CAD build for the part. Positions are in the model's coordinates, mm. Face numbers are marked on the shaded views. Coordinates: 2 decimals unless noted, no trailing zeros.
1) Pin check, flat tips, straight feed: pin 1 Ø1 at (y, z) = (-17.5, -1) entering from +X; pin 2 Ø1 at (x, z) = (19, 1) entering from +Y; pin 3 Ø1.5 at (x, z) = (6.5, -0.5) entering from -Y. Stop position of each tip, or through.
2) Two-plate mould, pull along X, no slides. Class the marked faces 1, 2 and 3: +X half, -X half, draft (parallel to the pull), parting line (faces both ways), or undercut.
3) Wall check: line 1 along X through (y, z) = (-8, 0.55); line 2 along X through (y, z) = (-7, -0.7); line 3 along Y through (x, z) = (-18.36, 0.7). Give the ranges that are in metal, low to high.
4) Saw through at A-A, the plane z = -0.5. Give the number of separate pieces and of enclosed holes in the cut face, and give its area (3 significant figures).
```python
from build123d import *

# Parameters (mm, degrees)
BOSS_EXTRUDE1_DEPTH  = 1.5875
M4_CLEARANCE_HOLE1_D = 4.5
BOSS_EXTRUDE2_DEPTH  = 3.175
FILLET1_R            = 3.5
M3_CLEARANCE_HOLE1_D = 3.4
SKETCH8_R            = 4
CUT_EXTRUDE1_DEPTH   = 4.1750001


with BuildPart() as part:
    # Sketch2 → Boss-Extrude1 (new body, symmetric)
    with BuildSketch(Plane.XY):
        with BuildLine():
            ThreePointArc((-17.942568571, -13.649816766), (-25.009816766, -13.417431429), (-24.777431429, -6.350183234))
            add(Edge.make_bspline(
                [(-24.777431429, -6.350183234), (-20.441430485, -2.271315687), (-12.829947979, 2.196277878), (-6.501150321, 4.42663028), (0, 5.19112324), (6.501150321, 4.42663028), (12.829947979, 2.196277878), (20.441430485, -2.271315687), (24.777431429, -6.350183234)],
                knots=[0, 0, 0, 0.1875, 0.3125, 0.4375, 0.5625, 0.6875, 0.8125, 1, 1, 1], degree=2))
            ThreePointArc((24.777431429, -6.350183234), (25.009816766, -13.417431429), (17.942568571, -13.649816766))
            add(Edge.make_bspline(
                [(-17.942568571, -13.649816766), (-14.268569515, -10.228684313), (-8.530052021, -6.883777878), (-4.178849679, -5.36413028), (0, -4.87862324), (4.178849679, -5.36413028), (8.530052021, -6.883777878), (14.268569515, -10.228684313), (17.942568571, -13.649816766)],
                knots=[0, 0, 0, 0.1875, 0.3125, 0.4375, 0.5625, 0.6875, 0.8125, 1, 1, 1], degree=2))
        make_face()
    extrude(amount=BOSS_EXTRUDE1_DEPTH, both=True)

    # M4 Clearance Hole1 (through all)
    with Locations(Plane.XY.offset(1.5875)):
        with Locations((21.36, -10), (0, 0)):
            Hole(M4_CLEARANCE_HOLE1_D / 2)

    # Sketch5 → Boss-Extrude2 (add)
    with BuildSketch(Plane(origin=(0, 0, -1.5875), x_dir=(-1, 0, 0), z_dir=(0, 0, -1))):
        with BuildLine():
            ThreePointArc((13.518770817, -20.368950039), (17.11, -26.460179221), (23.201229183, -22.868950039))
            Line((23.201229183, -22.868950039), (26.201229183, -11.25))
            ThreePointArc((26.201229183, -11.25), (22.61, -5.158770817), (16.518770817, -8.75))
            Line((16.518770817, -8.75), (13.518770817, -20.368950039))
        make_face()
    extrude(amount=-BOSS_EXTRUDE2_DEPTH)

    # Fillet1
    fillet1_edges = [part.edges().sort_by_distance(p)[0] for p in [
        (-15.752223744, -11.718824048, 0.7937488),
    ]]
    fillet(fillet1_edges, radius=FILLET1_R)

    # M3 Clearance Hole1 (through all)
    with Locations(Plane(origin=(0, 0, -1.5875), x_dir=(-1, 0, 0), z_dir=(0, 0, -1))):
        with Locations((18.36, -21.618950039)):
            Hole(M3_CLEARANCE_HOLE1_D / 2)

    # Sketch8 → Cut-Extrude1 (cut, through all)
    with BuildSketch(Plane(origin=(0, 0, -1.5875), x_dir=(-1, 0, 0), z_dir=(0, 0, -1))):
        with Locations((21.36, -10)):
            Circle(SKETCH8_R)
    extrude(amount=-CUT_EXTRUDE1_DEPTH, mode=Mode.SUBTRACT)


solid = part.part
```
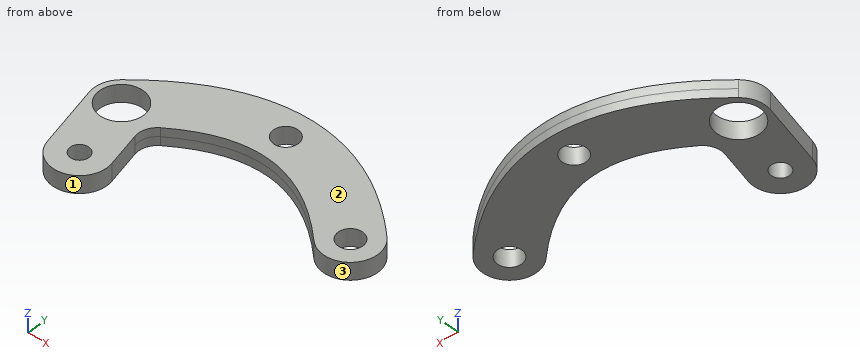
Data:
1. pin 1: stops at x = -14.13
1. pin 2: stops at y = -1.26
1. pin 3: stops at y = -6.46
2. face 1: parting line
2. face 2: draft
2. face 3: undercut
3. line 1: x = -25.94 to -24.82, -17.9 to -10.44, 10.44 to 20.33, 22.39 to 25.94
3. line 2: x = -25.36 to -24.01, -18.71 to -8.5, 8.5 to 25.36
3. line 3: y = -26.62 to -23.32, -19.92 to -12.65, -7.35 to -1.16
4. separate pieces: 1
4. enclosed holes: 4
4. area: 590 mm2
